from build123d import *

# Parameters (mm, degrees)
SKETCH1_W           = 220
SKETCH1_H           = 220
SKETCH1_R           = 10
BOSS_EXTRUDE2_DEPTH = 20
FILLET5_R           = 10
SKETCH6_R           = 102.5
BOSS_EXTRUDE3_DEPTH = 200


with BuildPart() as part:
    # Sketch1 → Boss-Extrude2 (new body)
    with BuildSketch(Plane(origin=(0, 0, 0), x_dir=(1, 0, 0), z_dir=(0, 1, 0))):
        Rectangle(SKETCH1_W, SKETCH1_H)
        with Locations(Location((-95, 95, 0), (0, 0, 270))):
            Circle(SKETCH1_R, mode=Mode.SUBTRACT)
        with Locations(Location((95, 95, 0), (0, 0, 270))):
            Circle(SKETCH1_R, mode=Mode.SUBTRACT)
        with Locations(Location((95, -95, 0), (0, 0, 270))):
            Circle(SKETCH1_R, mode=Mode.SUBTRACT)
        with Locations(Location((-95, -95, 0), (0, 0, 270))):
            Circle(SKETCH1_R, mode=Mode.SUBTRACT)
    extrude(amount=BOSS_EXTRUDE2_DEPTH)

    # Fillet5
    fillet5_edges = [part.edges().sort_by_distance(p)[0] for p in [
        (110, 10, 110),
        (-110, 10, 110),
        (-110, 10, -110),
        (110, 10, -110),
    ]]
    fillet(fillet5_edges, radius=FILLET5_R)

    # Sketch6 → Boss-Extrude3 (add)
    with BuildSketch(Plane(origin=(0, 20, 0), x_dir=(1, 0, 0), z_dir=(0, 1, 0))):
        with Locations(Location((0, 0, 0), (0, 0, 270))):
            Circle(SKETCH6_R)
    extrude(amount=BOSS_EXTRUDE3_DEPTH)


solid = part.part
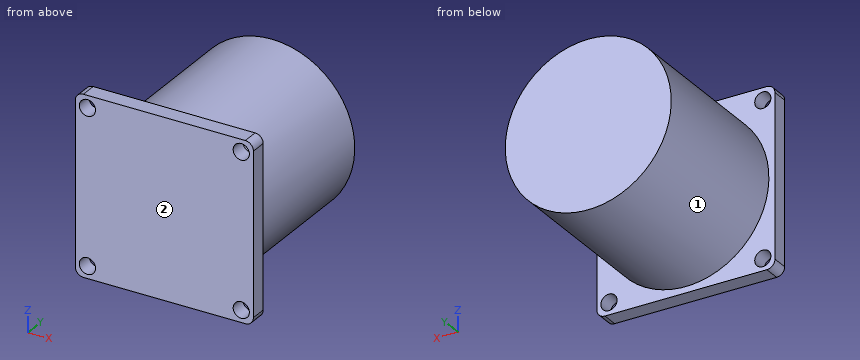
The listing builds one solid part. Answer for the finished solid, in the listing's coordinates (mm). Face numbers are marked on the shaded views. A direction names the side the tool comes from. Coordinates: 2 decimals unless noted, no trailing zeros. Loops run counter-clockwise (first coordinate to the right, second up) from the corner with the lowest first, then second, coordinate; pieces in that order, holes last. Notation, with made-up numbers: (27, 62.25) -> (41, 62.25) arc R21 cw to (41, 72.25) -> close; hole circle Ø1 at (6.25, 17). An arc over 180 degrees is marked (long way). Answer in a Markdown table with one row per item. Add a question column.
1. The part is cut by section D-D, the plane x = 23. Write down the section's boundary in (y, z).
2. Consider line 1 (X direction, y = 10.5, z = -95); line 2 (Y direction, x = 78.5, z = 98); line 3 (Z direction, x = 24, y = 86). Determine where each line is inside the solid, lowest interval first. Write a range as [from, to].
3. The part is cut by section A-A, the plane z = 95. Write down the section's boundary in (x, y).
4. Flat-ended cylindrical pins translate along their axes: P1, Ø2, axis at y = 175.5, z = -24, coming from the +X side; P2, Ø2, axis at x = -60.5, z = 20, coming from the -Y side; P3, Ø6, axis at y = 51, z = -65.5, coming from the +X side; P4, Ø6, axis at x = 40.5, y = 73.5, coming from the +Z side. Find the tip coordinate at first contact, or state that the pin passes through.
5. The part is cut by section B-B, the plane x = 95. Write down the section's boundary in (y, z).
6. For the marked faces 1 and 2, determine the directions among +Z, -Z, +X, -X, +Y, -Y from which every point of the face is accessible in a straight line to the end or side of a thin tool.
7. The part is cut by section C-C, the plane z = 0. Write down the section's boundary in (x, y).
Answer below:
| question | item | result |
|---|---|---|
| 1 | outline | (0, -110) -> (20, -110) -> (20, -99.89) -> (220, -99.89) -> (220, 99.89) -> (20, 99.89) -> (20, 110) -> (0, 110) -> close |
| 2 | line 1 | [-110, -105], [-85, 85], [105, 110] |
| 2 | line 2 | [0, 20] |
| 2 | line 3 | [-99.65, 99.65] |
| 3 | outline | (-110, 0) -> (-105, 0) -> (-105, 20) -> (-110, 20) -> close; (-85, 0) -> (85, 0) -> (85, 20) -> (38.49, 20) -> (38.49, 220) -> (-38.49, 220) -> (-38.49, 20) -> (-85, 20) -> close; (105, 0) -> (110, 0) -> (110, 20) -> (105, 20) -> close |
| 4 | P1 | x = 99.89 |
| 4 | P2 | y = 0 |
| 4 | P3 | x = 81.24 |
| 4 | P4 | z = 95.39 |
| 5 | outline | (0, -110) -> (20, -110) -> (20, -105) -> (0, -105) -> close; (0, -85) -> (20, -85) -> (20, -38.49) -> (220, -38.49) -> (220, 38.49) -> (20, 38.49) -> (20, 85) -> (0, 85) -> close; (0, 105) -> (20, 105) -> (20, 110) -> (0, 110) -> close |
| 6 | face 1 | +Y |
| 6 | face 2 | +Z, -Z, +X, -X, -Y |
| 7 | outline | (-110, 0) -> (110, 0) -> (110, 20) -> (102.5, 20) -> (102.5, 220) -> (-102.5, 220) -> (-102.5, 20) -> (-110, 20) -> close |
